Geometry: final body of the model. Coordinates: model frame, mm. A direction names the side the tool comes from. Coordinates: 2 decimals unless noted, no trailing zeros. Write each loop counter-clockwise with the first axis right and the second up, starting at its lowest first coordinate (ties: lowest second). Pieces come first, ordered by that corner, then holes.
from build123d import *

# Parameters (mm, degrees)
F1_DEPTH      = 600
F1_DEPTH_BACK = 600
F3_DEPTH      = 25
F3_DEPTH_BACK = 25


with BuildPart() as f1:
    # F0 (on Right) → F1 (new body, two sides)
    with BuildSketch(Plane.YZ) as f1_sk:
        with BuildLine():
            ThreePointArc((-20, -28), (-19.4142135624, -29.4142135624), (-18, -30))
            Line((-18, -30), (18, -30))
            ThreePointArc((18, -30), (19.4142135624, -29.4142135624), (20, -28))
            Line((20, -28), (20, 28))
            ThreePointArc((20, 28), (19.4142135624, 29.4142135624), (18, 30))
            Line((18, 30), (-18, 30))
            ThreePointArc((-18, 30), (-19.4142135624, 29.4142135624), (-20, 28))
            Line((-20, 28), (-20, -28))
        make_face()
        with BuildLine():
            Line((17, -28), (-17, -28))
            ThreePointArc((-17, -28), (-17.7071067812, -27.7071067812), (-18, -27))
            Line((-18, -27), (-18, 27))
            ThreePointArc((-18, 27), (-17.7071067812, 27.7071067812), (-17, 28))
            Line((-17, 28), (17, 28))
            ThreePointArc((17, 28), (17.7071067812, 27.7071067812), (18, 27))
            Line((18, 27), (18, -27))
            ThreePointArc((18, -27), (17.7071067812, -27.7071067812), (17, -28))
        make_face(mode=Mode.SUBTRACT)
    extrude(amount=F1_DEPTH)
    extrude(f1_sk.sketch, amount=-F1_DEPTH_BACK)

    # F2 (on Front) → F3 (cut, two sides)
    with BuildSketch(Plane.XZ) as f3_sk:
        Polygon((-600, 30), (-600, -30), (-540, 30), align=None)
        Polygon((540, 30), (600, -30), (600, 30), align=None)
    extrude(amount=-F3_DEPTH, mode=Mode.SUBTRACT)
    extrude(f3_sk.sketch, amount=F3_DEPTH_BACK, mode=Mode.SUBTRACT)


solid = f1.part
Item 1: Pull-direction query (Z, two-part tool) for faces 1 (the flat face through (8, -20, 0)), 2 (the flat face through (8, 0, 28)), 3 (the flat face through (8, 0, -30)); classes: released by +Z, released by -Z, zero draft, split by the parting line, or undercut.
Derived:
face 1: zero draft
face 2: undercut
face 3: released by -Z
Item 2: Section A-A, the plane z = -17.5. Output: boundary loops of the cut face in (x, y), plus the area to 3 significant figures.
Derived:
outline: (-587.5, -20) - (587.5, -20) - (587.5, -18) - (-587.5, -18) - close; (-587.5, 18) - (587.5, 18) - (587.5, 20) - (-587.5, 20) - close
area: 4,700 mm2
Item 3: Set-up query: faces 4 (the flat face through (8, -18, 0)), 5 (the flat face through (-572, -19, -2)). Return all of +Z, -Z, +X, -X, +Y, -Y with unobstructed straight access to the full face (end or side cutting, diameter ignored); none if empty.
Derived:
face 4: +X, -X
face 5: +Z, -X, +Y, -Y
Item 4: Section B-B, the plane y = 10. Output: boundary loops of the cut face in (x, z), plus the area to 3 significant figures.
Derived:
outline: (-600, -30) - (600, -30) - (598, -28) - (-598, -28) - close; (-542, 28) - (542, 28) - (540, 30) - (-540, 30) - close
area: 4,560 mm2
Item 5: Pin query (flat end, axial travel): pin 1 (6 mm diameter, centred on y = 13, z = 2.5, fed in from -X). Return the tip coordinate at first contact, or that it passes through.
Derived:
pin 1: passes through
Item 6: Section C-C, the plane x = 218. Output: boundary loops of the cut face in (y, z).
Derived:
outline: (-20, -28) arc R2 ccw to (-18, -30) - (18, -30) arc R2 ccw to (20, -28) - (20, 28) arc R2 ccw to (18, 30) - (-18, 30) arc R2 ccw to (-20, 28) - close; hole (-18, -27) arc R1 ccw to (-17, -28) - (17, -28) arc R1 ccw to (18, -27) - (18, 27) arc R1 ccw to (17, 28) - (-17, 28) arc R1 ccw to (-18, 27) - close
Item 7: Material intervals for probe 1 along Y at (x, z) = (-48.5, -2); probe 2 along Z at (x, y) = (-215, 15.5); probe 3 along X at (y, z) = (-18, 27.5), sorted ascending.
Derived:
probe 1: y = -20 to -18, 18 to 20
probe 2: z = -30 to -28, 28 to 30
probe 3: x = -542.5 to 542.5
